```python
from build123d import *

# Parameters (mm, degrees)
F0_W     = 6.35
F0_H     = 28.575
F1_DEPTH = 28.448
F2_DEPTH = 6.35
F3_DEPTH = 6.35
F4_DEPTH = 6.35
F5_DEPTH = 5.588
F6_DEPTH = 6.35
F7_DEPTH = 11.176
F8_DEPTH = 1.524


with BuildPart() as f1:
    # F0 (on Front) → F1 (new body)
    with BuildSketch(Plane.XZ):
        with Locations((-61.201207, 14.2875)):
            Rectangle(F0_W, F0_H)
        Polygon((5.219793, 28.575), (-58.026207, 28.575), (-58.026207, 0), (9.029793, 0), (11.696793, 0), (22.745793, 11.049), (5.219793, 11.049), align=None)
        with BuildLine():
            ThreePointArc((-44.21325, 9.054515), (-48.90092, 13.742185), (-44.21325, 18.429855))
            Line((-44.21325, 18.429855), (-11.399561, 18.429855))
            ThreePointArc((-11.399561, 18.429855), (-6.701007, 14.040749), (-10.760333, 9.054515))
            Line((-10.760333, 9.054515), (-44.21325, 9.054515))
        make_face(mode=Mode.SUBTRACT)
        Polygon((-58.026207, 0), (-64.376207, 0), (-64.376207, -31.75), (-58.026207, -31.75), (9.029793, -31.75), (9.029793, 0), align=None)
        Polygon((40.271793, 28.575), (5.219793, 28.575), (5.219793, 11.049), (22.745793, 11.049), align=None)
        with Locations((-61.201207, -46.0375)):
            Rectangle(F0_W, F0_H)
        Polygon((9.029793, -31.75), (-58.026207, -31.75), (-58.026207, -60.325), (5.219793, -60.325), (5.219793, -42.799), (22.745793, -42.799), (11.696793, -31.75), align=None)
        with BuildLine():
            ThreePointArc((-41.869413, -52.950572), (-47.864406, -48.643555), (-42.934794, -43.14908))
            Line((-42.934794, -43.14908), (-9.268802, -43.14908))
            ThreePointArc((-9.268802, -43.14908), (-4.368056, -48.049826), (-9.268802, -52.950572))
            Line((-9.268802, -52.950572), (-41.869413, -52.950572))
        make_face(mode=Mode.SUBTRACT)
        Polygon((5.219793, -42.799), (5.219793, -60.325), (40.271793, -60.325), (22.745793, -42.799), align=None)
    extrude(amount=-F1_DEPTH)

    # F0 (on Front) → F2 (cut)
    with BuildSketch(Plane.XZ):
        Polygon((5.219793, 28.575), (-58.026207, 28.575), (-58.026207, 0), (9.029793, 0), (11.696793, 0), (22.745793, 11.049), (5.219793, 11.049), align=None)
        with BuildLine():
            ThreePointArc((-44.21325, 9.054515), (-48.90092, 13.742185), (-44.21325, 18.429855))
            Line((-44.21325, 18.429855), (-11.399561, 18.429855))
            ThreePointArc((-11.399561, 18.429855), (-6.701007, 14.040749), (-10.760333, 9.054515))
            Line((-10.760333, 9.054515), (-44.21325, 9.054515))
        make_face(mode=Mode.SUBTRACT)
    extrude(amount=F2_DEPTH, mode=Mode.SUBTRACT)

    # F0 (on Front) → F3 (cut)
    with BuildSketch(Plane.XZ):
        Polygon((9.029793, -31.75), (-58.026207, -31.75), (-58.026207, -60.325), (5.219793, -60.325), (5.219793, -42.799), (22.745793, -42.799), (11.696793, -31.75), align=None)
        with BuildLine():
            ThreePointArc((-41.869413, -52.950572), (-47.864406, -48.643555), (-42.934794, -43.14908))
            Line((-42.934794, -43.14908), (-9.268802, -43.14908))
            ThreePointArc((-9.268802, -43.14908), (-4.368056, -48.049826), (-9.268802, -52.950572))
            Line((-9.268802, -52.950572), (-41.869413, -52.950572))
        make_face(mode=Mode.SUBTRACT)
    extrude(amount=F3_DEPTH, mode=Mode.SUBTRACT)

    # F0 (on Front) → F4 (cut)
    with BuildSketch(Plane.XZ):
        Polygon((5.219793, 28.575), (-58.026207, 28.575), (-58.026207, 0), (9.029793, 0), (11.696793, 0), (22.745793, 11.049), (5.219793, 11.049), align=None)
        with BuildLine():
            ThreePointArc((-44.21325, 9.054515), (-48.90092, 13.742185), (-44.21325, 18.429855))
            Line((-44.21325, 18.429855), (-11.399561, 18.429855))
            ThreePointArc((-11.399561, 18.429855), (-6.701007, 14.040749), (-10.760333, 9.054515))
            Line((-10.760333, 9.054515), (-44.21325, 9.054515))
        make_face(mode=Mode.SUBTRACT)
    extrude(amount=-F4_DEPTH, mode=Mode.SUBTRACT)

    # F0 (on Front) → F5 (cut, symmetric)
    with BuildSketch(Plane.XZ):
        Polygon((5.219793, 28.575), (-58.026207, 28.575), (-58.026207, 0), (9.029793, 0), (11.696793, 0), (22.745793, 11.049), (5.219793, 11.049), align=None)
        with BuildLine():
            ThreePointArc((-44.21325, 9.054515), (-48.90092, 13.742185), (-44.21325, 18.429855))
            Line((-44.21325, 18.429855), (-11.399561, 18.429855))
            ThreePointArc((-11.399561, 18.429855), (-6.701007, 14.040749), (-10.760333, 9.054515))
            Line((-10.760333, 9.054515), (-44.21325, 9.054515))
        make_face(mode=Mode.SUBTRACT)
        Polygon((9.029793, -31.75), (-58.026207, -31.75), (-58.026207, -60.325), (5.219793, -60.325), (5.219793, -42.799), (22.745793, -42.799), (11.696793, -31.75), align=None)
        with BuildLine():
            ThreePointArc((-41.869413, -52.950572), (-47.864406, -48.643555), (-42.934794, -43.14908))
            Line((-42.934794, -43.14908), (-9.268802, -43.14908))
            ThreePointArc((-9.268802, -43.14908), (-4.368056, -48.049826), (-9.268802, -52.950572))
            Line((-9.268802, -52.950572), (-41.869413, -52.950572))
        make_face(mode=Mode.SUBTRACT)
    extrude(amount=F5_DEPTH, both=True, mode=Mode.SUBTRACT)

    # F0 (on Front) → F6 (cut)
    with BuildSketch(Plane.XZ):
        Polygon((5.219793, 28.575), (-58.026207, 28.575), (-58.026207, 0), (9.029793, 0), (11.696793, 0), (22.745793, 11.049), (5.219793, 11.049), align=None)
        with BuildLine():
            ThreePointArc((-44.21325, 9.054515), (-48.90092, 13.742185), (-44.21325, 18.429855))
            Line((-44.21325, 18.429855), (-11.399561, 18.429855))
            ThreePointArc((-11.399561, 18.429855), (-6.701007, 14.040749), (-10.760333, 9.054515))
            Line((-10.760333, 9.054515), (-44.21325, 9.054515))
        make_face(mode=Mode.SUBTRACT)
        Polygon((9.029793, -31.75), (-58.026207, -31.75), (-58.026207, -60.325), (5.219793, -60.325), (5.219793, -42.799), (22.745793, -42.799), (11.696793, -31.75), align=None)
        with BuildLine():
            ThreePointArc((-41.869413, -52.950572), (-47.864406, -48.643555), (-42.934794, -43.14908))
            Line((-42.934794, -43.14908), (-9.268802, -43.14908))
            ThreePointArc((-9.268802, -43.14908), (-4.368056, -48.049826), (-9.268802, -52.950572))
            Line((-9.268802, -52.950572), (-41.869413, -52.950572))
        make_face(mode=Mode.SUBTRACT)
    extrude(amount=-F6_DEPTH, mode=Mode.SUBTRACT)

    # F0 (on Front) → F7 (cut)
    with BuildSketch(Plane.XZ):
        with Locations((-61.201207, 14.2875)):
            Rectangle(F0_W, F0_H)
        with Locations((-61.201207, -46.0375)):
            Rectangle(F0_W, F0_H)
    extrude(amount=-F7_DEPTH, mode=Mode.SUBTRACT)

    # F0 (on Front) → F8 (cut)
    with BuildSketch(Plane.XZ):
        Polygon((40.271793, 28.575), (5.219793, 28.575), (5.219793, 11.049), (22.745793, 11.049), align=None)
        Polygon((5.219793, -42.799), (5.219793, -60.325), (40.271793, -60.325), (22.745793, -42.799), align=None)
    extrude(amount=-F8_DEPTH, mode=Mode.SUBTRACT)


solid = f1.part
```
Geometry check sheet. Reference: the model listing, model coordinates, mm. A direction names the side the tool comes from. Coordinates: 2 decimals unless noted, no trailing zeros. Order: outer loops, then holes, each group sorted by start corner. A loop starts at its lowest first (then second) coordinate and runs counter-clockwise, first axis right, second up. Notation, with made-up numbers: (-13, 66) - (-8, 66) arc R20 ccw to (-8, 81) - close; hole circle Ø6 at (81, -30.5). An arc over 180 degrees is marked (long way). Answer in a Markdown table with one row per item. Add a question column.
1. Section check A-A (z = 13). Enter the section's corners in (x, y).
2. Section check C-C (x = 2.5). Enter the section's corners in (y, z) (3 decimals), plus the area to 3 significant figures.
3. Draft check along X on faces 1 (the face through (19, 1.524, -51)), 2 (the face through (25.784, 14.798, 14.087)), 3 (the face through (-58.026, 9, -46)), 4 (the face through (-48.9, 17.2, 13.6)). Enter one of: +X half, -X half, draft (parallel to the pull), parting line (faces both ways), or undercut.
4. Section check D-D (x = 13.5). Enter the section's corners in (y, z) (3 decimals), plus the area to 3 significant figures.
5. Section check B-B (y = 9.5). Give the number of separate pieces and of enclosed holes in the cut face, plus the area to 3 significant figures.
6. Access from +Z, -Z, +X, -X, +Y, -Y to the whole of each face (thin tool, end or side, straight path). Record for faces 5 (the face through (-61, 11.176, 14)), 6 (the face through (9.03, 14, -16)), 7 (the face through (14, 4, 11.049)), 8 (the face through (-28, 17, 18.43)), 9 (the face through (-61, 11.176, -46)).
7. Gauge pin test, flat ends, axial feed: pin 1 Ø4 at (y, z) = (9, 21) entering from -X; pin 2 Ø14.5 at (x, z) = (-6, -40.5) entering from -Y; pin 3 Ø14 at (x, z) = (16.5, 22) entering from -Y. Record the tip position at first contact, or that the pin passes through.
8. Material ranges on L1, parallel to Z at x = -37.5, y = 20 (3 decimals); L2, parallel to Z at x = -14, y = 2.75; L3, parallel to Y at x = -3.5, z = -54, recorded low to high. Write a range as [from, to].
Data:
| question | item | result |
|---|---|---|
| 1 | outline | (-64.38, 11.18) - (-58.03, 11.18) - (-58.03, 6.35) - (-48.84, 6.35) - (-48.84, 28.45) - (-64.38, 28.45) - close; (-6.75, 6.35) - (5.22, 6.35) - (5.22, 1.52) - (24.7, 1.52) - (24.7, 28.45) - (-6.75, 28.45) - close |
| 2 | outline | (0, -31.75) - (6.35, -31.75) - (6.35, -60.325) - (28.448, -60.325) - (28.448, 28.575) - (6.35, 28.575) - (6.35, 0) - (0, 0) - close |
| 2 | area | 2,170 mm² |
| 3 | face 1 | draft |
| 3 | face 2 | +X half |
| 3 | face 3 | -X half |
| 3 | face 4 | undercut |
| 4 | outline | (1.524, -60.325) - (28.448, -60.325) - (28.448, -33.553) - (6.35, -33.553) - (6.35, -42.799) - (1.524, -42.799) - close; (1.524, 11.049) - (6.35, 11.049) - (6.35, 1.803) - (28.448, 1.803) - (28.448, 28.575) - (1.524, 28.575) - close |
| 4 | area | 1,350 mm² |
| 5 | separate pieces | 1 |
| 5 | enclosed holes | 2 |
| 5 | area | 6,350 mm² |
| 6 | face 5 | +Z, -X, -Y |
| 6 | face 6 | +X, +Y, -Y |
| 6 | face 7 | +X, -X, -Y |
| 6 | face 8 | +Y, -Y |
| 6 | face 9 | -Z, -X, -Y |
| 7 | pin 1 | stops at x = -58.03 |
| 7 | pin 2 | stops at y = 6.35 |
| 7 | pin 3 | stops at y = 1.52 |
| 8 | L1 | z = [-60.325, -52.951], [-43.149, 9.055], [18.43, 28.575] |
| 8 | L2 | z = [-31.75, 0] |
| 8 | L3 | y = [6.35, 28.45] |
